Design review of the part built by this model. Coordinates are the model's own, in mm. A direction names the side the tool comes from. Coordinates: 2 decimals unless noted, no trailing zeros. Order: outer loops, then holes, each group sorted by start corner. A loop starts at its lowest first (then second) coordinate and runs counter-clockwise, first axis right, second up. Notation, with made-up numbers: M -1,-5.75 L 30,-5.75 A31 ccw 30,25.25 Z; hole C 27.25,-37 d5. An arc over 180 degrees is marked long. Answer as a JSON object with one key per item and string values.
from build123d import *

# Parameters (mm, degrees)
BOSS_EXTRUDE2_DEPTH = 12.5
SKETCH2_R           = 6
CUT_EXTRUDE1_DEPTH  = 59.662168388
FILLET1_RADIUS      = 12.5
FILLET1_LENGTH      = 5
FILLET2_RADIUS      = 12.5
FILLET2_LENGTH      = 5


with BuildPart() as part:
    # Sketch1 → Boss-Extrude2 (new, symmetric)
    with BuildSketch(Plane(origin=(0, 0, 0), x_dir=(0, 0, -1), z_dir=(1, 0, 0))):
        with BuildLine():
            Line((0, 5), (0, 11))
            Line((0, 11), (-18.857864376, 11))
            ThreePointArc((-18.857864376, 11), (-22.6846987, 10.238795325), (-25.928932188, 8.071067812))
            Line((-25.928932188, 8.071067812), (-26.071067812, 7.928932188))
            ThreePointArc((-26.071067812, 7.928932188), (-29.3153013, 5.761204675), (-33.142135624, 5))
            Line((-33.142135624, 5), (-57, 5))
            Line((-57, 5), (-57, 0))
            Line((-57, 0), (-31.071067812, 0))
            ThreePointArc((-31.071067812, 0), (-29.15765065, 0.380602337), (-27.535533906, 1.464466094))
            Line((-27.535533906, 1.464466094), (-25.464466094, 3.535533906))
            ThreePointArc((-25.464466094, 3.535533906), (-23.84234935, 4.619397663), (-21.928932188, 5))
            Line((-21.928932188, 5), (0, 5))
        make_face()
        with BuildLine():
            Line((18.857864376, 11), (0, 11))
            Line((0, 11), (0, 5))
            Line((0, 5), (21.928932188, 5))
            ThreePointArc((21.928932188, 5), (23.84234935, 4.619397663), (25.464466094, 3.535533906))
            Line((25.464466094, 3.535533906), (27.535533906, 1.464466094))
            ThreePointArc((27.535533906, 1.464466094), (29.15765065, 0.380602337), (31.071067812, 0))
            Line((31.071067812, 0), (57, 0))
            Line((57, 0), (57, 5))
            Line((57, 5), (33.142135624, 5))
            ThreePointArc((33.142135624, 5), (29.3153013, 5.761204675), (26.071067812, 7.928932188))
            Line((26.071067812, 7.928932188), (25.928932188, 8.071067812))
            ThreePointArc((25.928932188, 8.071067812), (22.6846987, 10.238795325), (18.857864376, 11))
        make_face()
    extrude(amount=BOSS_EXTRUDE2_DEPTH, both=True)

    # Sketch2 → Cut-Extrude1 (cut, through all)
    with BuildSketch(Plane(origin=(0, 5, 0), x_dir=(1, 0, 0), z_dir=(0, 1, 0))):
        with Locations(Location((0, 44.5, 0), (0, 0, 270))):
            Circle(SKETCH2_R)
        with Locations(Location((0, -44.5, 0), (0, 0, 90))):
            Circle(SKETCH2_R)
    extrude(amount=-CUT_EXTRUDE1_DEPTH, mode=Mode.SUBTRACT)

    # Fillet1: full round fillet: the end face becomes a half cylinder, R = half its width
    fillet1_face = Plane((0, 2.5, -57), x_dir=(0, 1, 0), z_dir=(0, 0, -1))  # on the end face: x along it, z out of the body
    fillet1_slab = fillet1_face.offset(-FILLET1_RADIUS / 2) * Box(FILLET1_LENGTH, 2 * FILLET1_RADIUS, FILLET1_RADIUS, mode=Mode.PRIVATE)  # the body's end, R deep
    fillet1_round = Plane((0, 2.5, -44.5), x_dir=(0, 0, -1), z_dir=(0, 1, 0)) * Cylinder(FILLET1_RADIUS, FILLET1_LENGTH, mode=Mode.PRIVATE)  # its axis R under the face
    add(fillet1_slab - fillet1_round, mode=Mode.SUBTRACT)

    # Fillet2: full round fillet: the end face becomes a half cylinder, R = half its width
    fillet2_face = Plane((0, 2.5, 57), x_dir=(0, -1, 0), z_dir=(0, 0, 1))  # on the end face: x along it, z out of the body
    fillet2_slab = fillet2_face.offset(-FILLET2_RADIUS / 2) * Box(FILLET2_LENGTH, 2 * FILLET2_RADIUS, FILLET2_RADIUS, mode=Mode.PRIVATE)  # the body's end, R deep
    fillet2_round = Plane((0, 2.5, 44.5), x_dir=(0, 0, 1), z_dir=(0, -1, 0)) * Cylinder(FILLET2_RADIUS, FILLET2_LENGTH, mode=Mode.PRIVATE)  # its axis R under the face
    add(fillet2_slab - fillet2_round, mode=Mode.SUBTRACT)


solid = part.part
1) Add section C-C (z = 5). State the section outline as (x, y) points.
Taken from the geometry:
{"outline": "M -12.5,5 L 12.5,5 L 12.5,11 L -12.5,11 Z"}
2) Mouldability with a two-part tool opening along Z and no side actions: class faces 4 (the cylindrical face through (0.18, 4.63, -23.82)), 5 (the flat face through (0, 11, 0)), 6 (the cylindrical face through (0.175, 10.218, -22.735)) as released by +Z, released by -Z, zero draft, split by the parting line, or undercut.
Taken from the geometry:
{"face 4": "undercut", "face 5": "zero draft", "face 6": "released by -Z"}
3) Add section D-D (x = 10.75). State the section outline as (y, z) points, and give its area (3 significant figures).
Taken from the geometry:
{"outline": "M 0,-50.88 L 5,-50.88 L 5,-33.14 A10 cw 7.93,-26.07 L 8.07,-25.93 A10 ccw 11,-18.86 L 11,18.86 A10 ccw 8.07,25.93 L 7.93,26.07 A10 cw 5,33.14 L 5,50.88 L 0,50.88 L 0,31.07 A5 ccw 1.46,27.54 L 3.54,25.46 A5 cw 5,21.93 L 5,-21.93 A5 cw 3.54,-25.46 L 1.46,-27.54 A5 ccw 0,-31.07 Z", "area": "556 mm2"}
4) Insertion check: pin 1 Ø2 at (x, z) = (-9.5, 25.5) entering from +Y; pin 2 Ø11 at (x, z) = (0, -44.5) entering from -Y; pin 3 Ø6 at (x, y) = (4.5, 6) entering from -Z; pin 4 Ø5 at (x, y) = (-8, 5) entering from -Z (3 decimals). Each pin has a flat end and moves straight along its axis. Give the tip position at first contact, or say it passes through.
Taken from the geometry:
{"pin 1": "stops at y = 9.26", "pin 2": "passes through", "pin 3": "stops at z = -56.89", "pin 4": "stops at z = -55.725"}
5) To check wall thickness, follow L1, parallel to Z at x = 5, y = 1.25; L2, parallel to X at y = 2.85, z = 44.5; L3, parallel to Z at x = 5, y = 3.5. State the ranges of each line that lie inside material, in increasing order.
Taken from the geometry:
{"L1": "z = -55.96 to -47.82, -41.18 to -27.76, 27.76 to 41.18, 47.82 to 55.96", "L2": "x = -12.5 to -6, 6 to 12.5", "L3": "z = -55.96 to -47.82, -41.18 to -25.5, 25.5 to 41.18, 47.82 to 55.96"}
6) Add section A-A (y = 2.5). State the section outline as (x, z) points.
Taken from the geometry:
{"outline": "M -12.5,-44.5 A12.5 ccw 12.5,-44.5 L 12.5,-26.5 L -12.5,-26.5 Z; M -12.5,26.5 L 12.5,26.5 L 12.5,44.5 A12.5 ccw -12.5,44.5 Z; hole C 0,-44.5 d12; hole C 0,44.5 d12"}
7) Add section B-B (x = 0). State the section outline as (y, z) points, and give its area (3 significant figures).
Taken from the geometry:
{"outline": "M 0,-57 L 5,-57 L 5,-50.5 L 0,-50.5 Z; M 0,-38.5 L 5,-38.5 L 5,-33.14 A10 cw 7.93,-26.07 L 8.07,-25.93 A10 ccw 11,-18.86 L 11,18.86 A10 ccw 8.07,25.93 L 7.93,26.07 A10 cw 5,33.14 L 5,38.5 L 0,38.5 L 0,31.07 A5 ccw 1.46,27.54 L 3.54,25.46 A5 cw 5,21.93 L 5,-21.93 A5 cw 3.54,-25.46 L 1.46,-27.54 A5 ccw 0,-31.07 Z; M 0,50.5 L 5,50.5 L 5,57 L 0,57 Z", "area": "497 mm2"}
8) Tool access review of faces 1 (the flat face through (6, 5, -43)), 2 (the cylindrical face through (0, 3, -57)), 3 (the flat face through (0, 3, -26)): name each direction out of +Z, -Z, +X, -X, +Y, -Y from which nothing blocks a thin tool from reaching the whole face with its end or side.
Taken from the geometry:
{"face 1": "-Z, +X, -X, +Y", "face 2": "-Z, +Y, -Y", "face 3": "+X, -X, -Y"}
